```python
from build123d import *

# Parameters (mm, degrees)
SKETCH1_R               = 5.75
BOSS_EXTRUDE1_DEPTH     = 18.5
BOSS_EXTRUDE2_DEPTH     = 29
CUT_EXTRUDE1_DEPTH      = 126.623445264
CUT_EXTRUDE2_DEPTH      = 122.581248554
FILLET1_R               = 3.5
CHAMFER1_SIZE           = 2
CUT_EXTRUDE3_DEPTH      = 119.245507314
CUT_EXTRUDE3_DEPTH_BACK = 119.245507314
SKETCH7_R               = 3.5
CUT_EXTRUDE4_DEPTH      = 10
CUT_EXTRUDE4_DEPTH_BACK = 1
SKETCH9_R               = 6
CUT_EXTRUDE5_DEPTH      = 10
FILLET3_R               = 3.5
CHAMFER2_SIZE           = 2
FILLET4_R               = 5


with BuildPart() as part:
    # Sketch1 → Boss-Extrude1 (new body)
    with BuildSketch(Plane(origin=(0, 0, 0), x_dir=(1, 0, 0), z_dir=(0, 1, 0))):
        with BuildLine():
            Line((-29, 50), (0, 50))
            ThreePointArc((0, 50), (22.285714286, 43.005420459), (36.577623382, 24.530612245))
            ThreePointArc((36.577623382, 24.530612245), (40.242215458, 19.793481934), (45.956501172, 18))
            Line((45.956501172, 18), (49, 18))
            Line((49, 18), (49, 13.5))
            Line((49, 13.5), (32.403703492, 13.5))
            ThreePointArc((32.403703492, 13.5), (-32.5, 11), (32.403703492, 8.5))
            Line((32.403703492, 8.5), (49, 8.5))
            Line((49, 8.5), (49, 4))
            Line((49, 4), (45.956501172, 4))
            ThreePointArc((45.956501172, 4), (40.242215458, 2.206518066), (36.577623382, -2.530612245))
            ThreePointArc((36.577623382, -2.530612245), (3.715197259, -27.822639134), (-33.347589544, -9.222222222))
            Line((-33.347589544, -9.222222222), (-33.594644376, -8.814814815))
            ThreePointArc((-33.594644376, -8.814814815), (-37.238774547, -5.286451588), (-42.145308361, -4))
            Line((-42.145308361, -4), (-46.173585522, -4))
            Line((-46.173585522, -4), (-74, -4))
            Line((-74, -4), (-105, -4))
            Line((-105, -4), (-105, 26))
            Line((-105, 26), (-74, 26))
            Line((-74, 26), (-52, 26))
            ThreePointArc((-52, 26), (-42.807611845, 29.807611845), (-39, 39))
            Line((-39, 39), (-39, 40))
            ThreePointArc((-39, 40), (-36.071067812, 47.071067812), (-29, 50))
        make_face()
        with Locations(Location((-30, 40, 0), (0, 0, 90))):
            Circle(SKETCH1_R, mode=Mode.SUBTRACT)
    extrude(amount=BOSS_EXTRUDE1_DEPTH)

    # Sketch3 → Boss-Extrude2 (add)
    with BuildSketch(Plane.XZ):
        Polygon((-105, -26), (-56, -26), (-56, -2.142135624), (-56, 4), (-105, 4), align=None)
    extrude(amount=BOSS_EXTRUDE2_DEPTH)

    # Sketch5 → Cut-Extrude1 (cut, through all)
    with BuildSketch(Plane(origin=(0, -29, 0), x_dir=(-1, 0, 0), z_dir=(0, -1, 0))):
        Polygon((66, 3.5), (66, 18.5), (105, 18.5), (105, 11), (105, 3.5), align=None)
    extrude(amount=-CUT_EXTRUDE1_DEPTH, mode=Mode.SUBTRACT)

    # Sketch6 → Cut-Extrude2 (cut, through all)
    with BuildSketch(Plane.XY.offset(4)):
        Polygon((-92, 11), (-100, 11), (-100, -26), (-92, -26), (-92, -5.5), align=None)
    extrude(amount=-CUT_EXTRUDE2_DEPTH, mode=Mode.SUBTRACT)

    # Fillet1
    fillet1_edges = [part.edges().sort_by_distance(p)[0] for p in [
        (-92, 11, -22.25),
        (-92, 11, 0.25),
        (-92, -26, -22.25),
        (-92, -26, 0.25),
        (-100, -26, -22.25),
        (-100, -26, 0.25),
        (-100, 11, -22.25),
        (-100, 11, 0.25),
        (-56, -29, -11),
        (-105, -29, 0.25),
        (-105, -29, -22.25),
    ]]
    fillet(fillet1_edges, radius=FILLET1_R)

    # Chamfer1
    chamfer1_edges = [part.edges().sort_by_distance(p)[0] for p in [
        (-105, 18.5, -22.25),
        (-105, 18.5, 0.25),
    ]]
    chamfer(chamfer1_edges, length=CHAMFER1_SIZE)

    # Sketch7 → Cut-Extrude3 (cut, two sides: drawn at the far end of the back side and taken through both)
    with BuildSketch(Plane.XY.offset(-4).offset(-CUT_EXTRUDE3_DEPTH_BACK)):
        with Locations(Location((42.5, 10, 0), (0, 0, 350.957402384))):
            Circle(SKETCH7_R)
    extrude(amount=CUT_EXTRUDE3_DEPTH + CUT_EXTRUDE3_DEPTH_BACK, mode=Mode.SUBTRACT)

    # Sketch8 → Cut-Extrude4 (cut, two sides: drawn at the far end of the back side and taken through both)
    with BuildSketch(Plane(origin=(0, 0, -18), x_dir=(-1, 0, 0), z_dir=(0, 0, -1)).offset(-CUT_EXTRUDE4_DEPTH_BACK)):
        Polygon((-42.5, 16.062177826), (-47.75, 13.031088913), (-47.75, 6.968911087), (-42.5, 3.937822174), (-37.25, 6.968911087), (-37.25, 13.031088913), align=None)
    extrude(amount=CUT_EXTRUDE4_DEPTH + CUT_EXTRUDE4_DEPTH_BACK, mode=Mode.SUBTRACT)

    # Sketch9 → Cut-Extrude5 (cut)
    with BuildSketch(Plane.XY.offset(-4)):
        with Locations((42.5, 10)):
            Circle(SKETCH9_R)
    extrude(amount=CUT_EXTRUDE5_DEPTH, mode=Mode.SUBTRACT)

    # Fillet3
    # the kernel refuses this fillet: 3.5 mm, written as the material it takes off along each edge
    with BuildSketch(Plane(origin=(49, 0, -26.75), x_dir=(0, 1, 0), z_dir=(0, 0, 1)), Plane(origin=(49, 0, -17.25), x_dir=(0, 1, 0), z_dir=(0, 0, 1))) as fillet3_piece_1:
        with BuildLine():
            CenterArc((FILLET3_R, FILLET3_R), FILLET3_R, 180, 90)
            Line((0, FILLET3_R), (0, 0))
            Line((0, 0), (FILLET3_R, 0))
        make_face()
    extrude(amount=22, mode=Mode.SUBTRACT)

    # Chamfer2
    chamfer2_edges = [part.edges().sort_by_distance(p)[0] for p in [
        (49, 18.5, -6.25),
        (49, 18.5, -15.75),
    ]]
    chamfer(chamfer2_edges, length=CHAMFER2_SIZE)

    # Fillet4
    fillet4_edges = [part.edges().sort_by_distance(p)[0] for p in [
        (-66, -5.25, -18.5),
        (-66, -5.25, -3.5),
    ]]
    fillet(fillet4_edges, radius=FILLET4_R)


solid = part.part
```
Geometry: final body of the model. Coordinates: model frame, mm. A direction names the side the tool comes from. Round coordinates to 2 decimals unless told otherwise and drop trailing zeros. Loops run counter-clockwise (first coordinate to the right, second up) from the corner with the lowest first, then second, coordinate; pieces in that order, holes last.
Item 1: Contact query for flat-ended pins moving along their axis: P1, Ø4, axis at y = 8.5, z = -9.5, coming from the +X side; P2, Ø13.5, axis at x = 44, y = 13.5, coming from the +Z side; P3, Ø10, axis at x = -88.5, y = -11, coming from the -Z side; P4, Ø2, axis at x = -89.5, y = -17.5, coming from the +Z side. Output: stop coordinate, or through.
Checked values:
P1: stops at x = 49
P2: stops at z = 1.08
P3: stops at z = -26
P4: stops at z = 4
Item 2: Section C-C, the plane x = 24. Output: boundary loops of the cut face in (y, z), plus the area to 3 significant figures.
Checked values:
outline: (0, -41.74) - (18.5, -41.74) - (18.5, -32.91) - (0, -32.91) - close; (0, 10.91) - (18.5, 10.91) - (18.5, 19.74) - (0, 19.74) - close
area: 327 mm2
Item 3: Line query: L1, parallel to Y at x = 42, z = -7; L2, parallel to X at y = 10, z = -15; L3, parallel to Z at x = -97, y = 14. Output: solid intervals per line, ascending.
Checked values:
L1: y = 0 to 6.54, 13.46 to 18.5
L2: x = -66.23 to -32.25, 32.25 to 39, 46 to 49
L3: z = -26 to -18.5, -3.5 to 4
Item 4: Section D-D, the plane z = -11. Output: boundary loops of the cut face in (x, y), plus the area to 3 significant figures.
Checked values:
outline: (-66, -29) - (-59.5, -29) arc R3.5 ccw to (-56, -25.5) - (-56, 0) - (-32.5, 0) - (-32.5, 18.5) - (-66, 18.5) - close
area: 907 mm2
Item 5: Reachability of faces 1 (the flat face through (-66, -6, -11)), 2 (the flat face through (45.162, 5.475, -17.617)), 3 (the cylindrical face through (-98.95, 10, 0.2)) from +Z, -Z, +X, -X, +Y, -Y: full face, straight path, thin tool, end or side. Return the list, or none.
Checked values:
face 1: -X, +Y, -Y
face 2: -Z
face 3: +Z, -Z
Item 6: Section B-B, the plane z = 1. Output: boundary loops of the cut face in (x, y).
Checked values:
outline: (-105, -25.5) arc R3.5 ccw to (-101.5, -29) - (-59.5, -29) arc R3.5 ccw to (-56, -25.5) - (-56, 0) - (-30.2, 0) - (-30.2, 18.5) - (-103, 18.5) - (-105, 16.5) - close; (30.2, 0) - (37.3, 0) - (37.3, 7.01) arc R6 cw to (37.3, 12.99) - (37.3, 18.5) - (30.2, 18.5) - close; hole (-100, -22.5) arc R3.5 ccw to (-96.5, -26) - (-95.5, -26) arc R3.5 ccw to (-92, -22.5) - (-92, 7.5) arc R3.5 ccw to (-95.5, 11) - (-96.5, 11) arc R3.5 ccw to (-100, 7.5) - close
Item 7: Mould query, pull axis X, two halves, no side actions, for faces 4 (the cylindrical face through (-57.05, -28, -10.79)), 5 (the cylindrical face through (-98.95, 10, -22.3)), 6 (the cylindrical face through (-42.909, 9.12, -29.707)). Classes: released by +X, released by -X, zero draft, split by the parting line, or undercut.
Checked values:
face 4: released by +X
face 5: undercut
face 6: released by -X
Item 8: Section A-A, the plane y = -19. Output: boundary loops of the cut face in (x, z).
Checked values:
outline: (-105, -26) - (-100, -26) - (-100, -18.5) - (-105, -18.5) - close; (-105, -3.5) - (-100, -3.5) - (-100, 4) - (-105, 4) - close; (-92, -26) - (-56, -26) - (-56, 4) - (-92, 4) - (-92, -3.5) - (-71, -3.5) arc R5 cw to (-66, -8.5) - (-66, -13.5) arc R5 cw to (-71, -18.5) - (-92, -18.5) - close
